Read the model definition and answer for the solid it produces. Units are mm, in the model's axes. Round coordinates to 2 decimals unless told otherwise and drop trailing zeros. Loops run counter-clockwise (first coordinate to the right, second up) from the corner with the lowest first, then second, coordinate; pieces in that order, holes last. Notation, with made-up numbers: M 56,-14.75 L 68,-14.75 A14 ccw 68,12.25 Z; hole C -35,-16 d9. An arc over 180 degrees is marked long. Write each question's results on one line, items separated by ' | '.
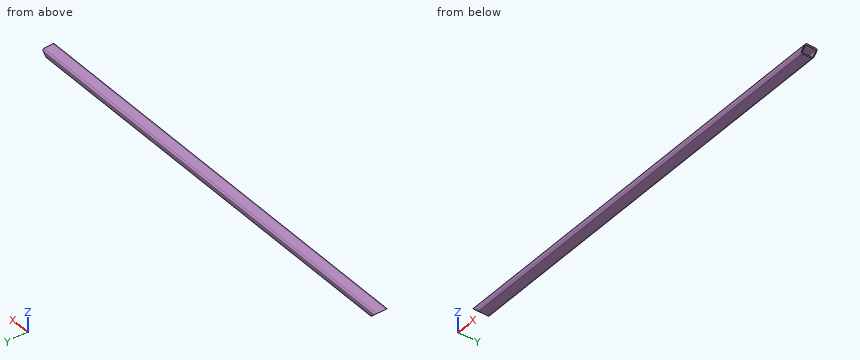
```python
from build123d import *

# Parameters (mm, degrees)
F1_DEPTH      = 431.8
F3_DEPTH      = 12.701
F3_DEPTH_BACK = 12.701


with BuildPart() as f1:
    # F0 (on Right) → F1 (new body, symmetric)
    with BuildSketch(Plane.YZ):
        with BuildLine():
            Line((-12.7, 3.175), (-12.7, -3.175))
            ThreePointArc((-12.7, -3.175), (-11.7700640303, -5.4200640303), (-9.525, -6.35))
            Line((-9.525, -6.35), (9.525, -6.35))
            ThreePointArc((9.525, -6.35), (11.7700640303, -5.4200640303), (12.7, -3.175))
            Line((12.7, -3.175), (12.7, 3.175))
            ThreePointArc((12.7, 3.175), (11.7700640303, 5.4200640303), (9.525, 6.35))
            Line((9.525, 6.35), (-9.525, 6.35))
            ThreePointArc((-9.525, 6.35), (-11.7700640303, 5.4200640303), (-12.7, 3.175))
        make_face()
        with BuildLine():
            ThreePointArc((-11.049, 3.175), (-10.6026307345, 4.2526307345), (-9.525, 4.699))
            Line((-9.525, 4.699), (9.525, 4.699))
            ThreePointArc((9.525, 4.699), (10.6026307345, 4.2526307345), (11.049, 3.175))
            Line((11.049, 3.175), (11.049, -3.175))
            ThreePointArc((11.049, -3.175), (10.6026307345, -4.2526307345), (9.525, -4.699))
            Line((9.525, -4.699), (-9.525, -4.699))
            ThreePointArc((-9.525, -4.699), (-10.6026307345, -4.2526307345), (-11.049, -3.175))
            Line((-11.049, -3.175), (-11.049, 3.175))
        make_face(mode=Mode.SUBTRACT)
    extrude(amount=F1_DEPTH, both=True)

    # F2 (on Front) → F3 (cut, two sides)
    with BuildSketch(Plane.XZ) as f3_sk:
        Polygon((-431.8, 6.35), (-431.8, -6.35), (-419.1, -6.35), align=None)
        Polygon((419.1, -6.35), (431.8, -6.35), (431.8, 6.35), align=None)
    extrude(amount=-F3_DEPTH, mode=Mode.SUBTRACT)
    extrude(f3_sk.sketch, amount=F3_DEPTH_BACK, mode=Mode.SUBTRACT)


solid = f1.part
```
1. Find the intervals of material crossed by L1, parallel to Y at x = 327.5, z = -0.25; L2, parallel to Z at x = -286.5, y = 7.5; L3, parallel to Z at x = -184, y = 10.25, in increasing order.
Completed:
L1: y = -12.7 to -11.05, 11.05 to 12.7 | L2: z = -6.35 to -4.7, 4.7 to 6.35 | L3: z = -6.27 to -4.52, 4.52 to 6.27
2. Given P1, Ø1, axis at y = 9.5, z = -2.5, coming from the -X side, flat-ended and moving along its own axis, determine where the tip first touches the part or whether it passes through.
Completed:
P1: passes through
3. Find section B-B, the plane z = 0.25. Give the vertices of the cut face in (x, y).
Completed:
outline: M -425.7,-12.7 L 425.7,-12.7 L 425.7,-11.05 L -425.7,-11.05 Z; M -425.7,11.05 L 425.7,11.05 L 425.7,12.7 L -425.7,12.7 Z
4. Find section C-C, the plane x = -305. Give the vertices of the cut face in (y, z) (3 decimals), then the cut area to 3 significant figures.
Completed:
outline: M -12.7,-3.175 A3.175 ccw -9.525,-6.35 L 9.525,-6.35 A3.175 ccw 12.7,-3.175 L 12.7,3.175 A3.175 ccw 9.525,6.35 L -9.525,6.35 A3.175 ccw -12.7,3.175 Z; hole M -11.049,-3.175 A1.524 ccw -9.525,-4.699 L 9.525,-4.699 A1.524 ccw 11.049,-3.175 L 11.049,3.175 A1.524 ccw 9.525,4.699 L -9.525,4.699 A1.524 ccw -11.049,3.175 Z | area: 108 mm2
5. Find section A-A, the plane y = -4.75. Give the vertices of the cut face in (x, z), then the cut area to 3 significant figures.
Completed:
outline: M -431.8,6.35 L -430.15,4.7 L 430.15,4.7 L 431.8,6.35 Z; M -420.75,-4.7 L -419.1,-6.35 L 419.1,-6.35 L 420.75,-4.7 Z | area: 2,810 mm2
